Geometry: final body of the model. Coordinates: model frame, mm. Face numbers are marked on the shaded views. A direction names the side the tool comes from. Give positions to 0.01 mm unless a question says otherwise; leave off trailing zeros. Loops run counter-clockwise (first coordinate to the right, second up) from the corner with the lowest first, then second, coordinate; pieces in that order, holes last. Notation, with made-up numbers: (-19, 46.25) -> (38, 46.25) arc R17 cw to (38, 57.25) -> close; hole circle Ø5 at (19.25, 27). An arc over 180 degrees is marked (long way). Answer in a Markdown table with one row per item. Add a question column.
1) Section query B-B (z = 0). Give the number of separate pieces and of enclosed holes in the cut face, plus the area to 3 significant figures.
2) Draft query along X for the marked faces 1 and 2. Return one class per face: +X half, -X half, draft (parallel to the pull), parting line (faces both ways), or undercut.
3) Access query for the marked faces 3 and 4. Directions: +Z, -Z, +X, -X, +Y, -Y. A direction counts if a zero-diameter tool reaches every point of the face in a straight line with its end or side. Return the directions, or none.
4) Section query A-A (x = 19.25). Return the cut outline in (y, z).
5) Line query: line 1 (Y direction, x = -3, z = 4.5); line 2 (Z direction, x = 19.25, y = 0.7); line 3 (X direction, y = 10.5, z = -3). Output: solid intervals per line, ascending. Write a range as from..to.
6) First-contact query: P1, Ø6, axis at x = -0.5, y = 12.5, coming from the +Z side; P2, Ø6.5, axis at x = 19.25, z = 0, coming from the +Y side; P3, Ø3, axis at y = 3, z = 5.5, coming from the -X side. Flat tips, straight axial feed; report the tip coordinate or a pass-through.
Autodesk Inventor part; units mm, degrees
ref_plane "YZ Plane" through (0, 0, 0) normal (1, 0, 0) x (0, 1, 0)
ref_plane "XZ Plane" through (0, 0, 0) normal (0, 1, 0) x (-1, 0, 0)
ref_plane "XY Plane" through (0, 0, 0) normal (0, 0, 1) x (1, 0, 0)
sketch "Sketch1" plane through (0, 0, 0) normal (0, 1, 0) x (-1, 0, 0)
  circle A0 centre (19.25, 0) radius 2
  line L0 (0, 16) -> (0, -26.1596) construction
  arc A1 (22.026, -3.8544) -> (22.026, 3.8544) centre (19.25, 0) ccw
  line L1 (22.026, -3.8544) -> (9.3506, -12.9833)
  line L2 (22.026, 3.8544) -> (9.3506, 12.9833)
  line L3 (0, 0) -> (7.2695, 0) construction
  circle A2 centre (-19.25, 0) radius 2
  arc A3 (-22.026, 3.8544) -> (-22.026, -3.8544) centre (-19.25, 0) ccw
  line L4 (-22.026, -3.8544) -> (-9.3506, -12.9833)
  line L5 (-22.026, 3.8544) -> (-9.3506, 12.9833)
  arc A4 (9.3506, 12.9833) -> (-9.3506, 12.9833) centre (0, 0) ccw
  arc A5 (-9.3506, -12.9833) -> (9.3506, -12.9833) centre (0, 0) ccw
  point P0 (-7.2695, 0)
  dimension "d1" = 4
  dimension "d3" = 38.5
  dimension "d6" = 48
  dimension "d9" = 16
  dimension "d10" = 16
extrude "Extrusion1" add sketch "Sketch1" along normal blind 1
sketch "Sketch3" plane through (0, 0, 0) normal (0, 0, 1) x (1, 0, 0)
  line L0 (-17.25, 0) -> (-17.25, 1)
  line L1 (-17.25, 1) -> (17.25, 1)
  line L2 (17.25, 1) -> (17.25, 0)
  line L3 (17.25, 0) -> (-17.25, 0)
  line L4 (24, 1) -> (24, 0)
  line L5 (24, 0) -> (21.25, 0)
  line L6 (21.25, 0) -> (21.25, 1)
  line L7 (21.25, 1) -> (24, 1)
  line L8 (-24, 0) -> (-24, 1)
  line L9 (-24, 1) -> (-21.25, 1)
  line L10 (-21.25, 1) -> (-21.25, 0)
  line L11 (-21.25, 0) -> (-24, 0)
  line L12 (0, 1) -> (0, 13.5844) construction
  line L13 (9.3506, 1) -> (-9.3506, 1)
  arc A0 (-9.5, 16) -> (-15.5, 1) centre (6.25, 1) ccw
  line L14 (-9.5, 16) -> (-7, 16)
  line L15 (-7, 16) -> (-7, 1)
  line L16 (-7, 1) -> (-15.5, 1)
  line L17 (-22.026, 1) -> (-9.3506, 1)
  point P0 (0, 0)
  dimension "d11" = 31
  dimension "d12" = 16
  dimension "d13" = 19
  dimension "d14" = 14
revolve "Revolution1" add sketch "Sketch3" angle 360 about axis through (0, 1, 0) along (0, 1, 0) contours A0 L14 L15 L1
equation "\"d10\" = d9"
properties part number "caster_wheel_v5_base"
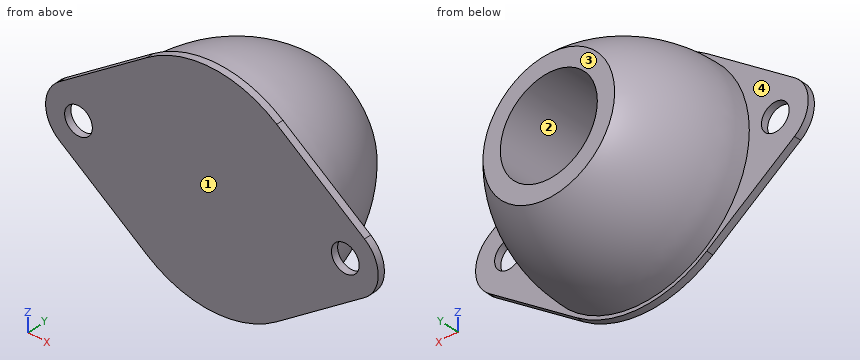
Evaluation:
| question | item | result |
|---|---|---|
| 1 | separate pieces | 3 |
| 1 | enclosed holes | 0 |
| 1 | area | 239 mm² |
| 2 | face 1 | draft |
| 2 | face 2 | undercut |
| 3 | face 3 | +Z, -Z, +X, -X, +Y |
| 3 | face 4 | +Y |
| 4 | outline | (0, -5.85) -> (1, -5.85) -> (1, -2) -> (0, -2) -> close; (0, 2) -> (1, 2) -> (1, 5.85) -> (0, 5.85) -> close |
| 5 | line 1 | 0..1 |
| 5 | line 2 | -5.85..-2, 2..5.85 |
| 5 | line 3 | -12.97..-6.32, 6.32..12.97 |
| 6 | P1 | z = 13.76 |
| 6 | P2 | y = 1 |
| 6 | P3 | x = -14.9 |
